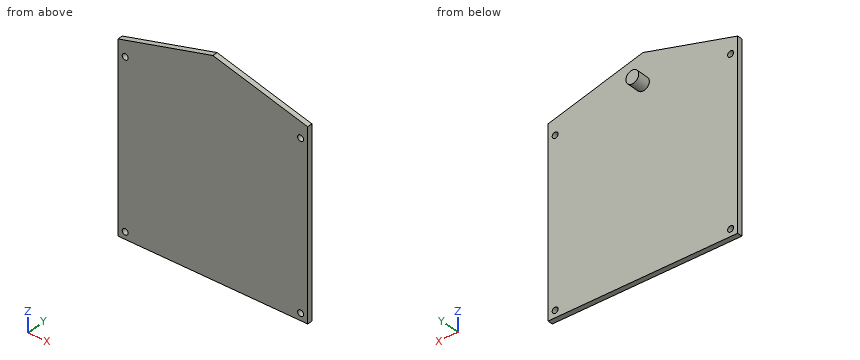
```python
from build123d import *

# Parameters (mm, degrees)
PAD_DEPTH    = 4
SKETCH001_R  = 2.3
POCKET_DEPTH = 5
SKETCH002_R  = 5
PAD001_DEPTH = 10


with BuildPart() as part:
    # Sketch → Pad (new body)
    with BuildSketch(Plane.XZ):
        Polygon((0, 0), (147, 0), (147, 143.135135), (73.5, 163), (0, 143.135135), align=None)
    extrude(amount=PAD_DEPTH)

    # Sketch001 (on Face7 of Pad) → Pocket (cut)
    with BuildSketch(Plane.XZ.offset(4)):
        with Locations((5.5, 5.5)):
            Circle(SKETCH001_R)
        with Locations((141.5, 5.5)):
            Circle(SKETCH001_R)
        with Locations((141.5, 132.5)):
            Circle(SKETCH001_R)
        with Locations((5.5, 132.5)):
            Circle(SKETCH001_R)
    extrude(amount=-POCKET_DEPTH, mode=Mode.SUBTRACT)

    # Sketch002 (on Face4 of Pocket) → Pad001 (join)
    with BuildSketch(Plane(origin=(0, 0, 0), x_dir=(1, 0, 0), z_dir=(0, 1, 0))):
        with Locations((73.5, -140)):
            Circle(SKETCH002_R)
    extrude(amount=PAD001_DEPTH)


solid = part.part
```
Geometry: final body of the model. Coordinates: model frame, mm. Give positions to 0.01 mm unless a question says otherwise; leave off trailing zeros. Loops run counter-clockwise (first coordinate to the right, second up) from the corner with the lowest first, then second, coordinate; pieces in that order, holes last. Notation, with made-up numbers: (-31, 28) - (17, 28) arc R14 ccw to (17, 43) - close; hole circle Ø3 at (52, 37). An arc over 180 degrees is marked (long way). Answer as CSV lines item,"result". Start each with the question number.
(1) Pin query (flat end, axial travel): P1, Ø4, axis at x = 141.5, z = 132.5, coming from the -Y side; P2, Ø2, axis at x = 129, z = 86.5, coming from the +Y side; P3, Ø3, axis at x = 71, y = 1, coming from the +Z side. Return the tip coordinate at first contact, or that it passes through.
(2) Ray query, line 1 along X through (y, z) = (-1.85, 132.5); line 2 along Z through (x, y) = (141.5, -2); line 3 along Y through (x, z) = (15.5, 80.5). Return the intervals inside material, ascending. Write a range as [from, to].
(3) Section query C-C (y = 7.5). Output: boundary loops of the cut face in (x, z).
(4) Section query A-A (z = 132.5). Output: boundary loops of the cut face in (x, y).
(5) Section query B-B (x = 141.5). Output: boundary loops of the cut face in (y, z), and give its area (3 significant figures).
(6) Section query D-D (z = 149). Output: boundary loops of the cut face in (x, y).
Worked answers:
1,P1,"passes through"
1,P2,"stops at y = 0"
1,P3,"stops at z = 162.63"
2,line 1,"x = [0, 3.2], [7.8, 139.2], [143.8, 147]"
2,line 2,"z = [0, 3.2], [7.8, 130.2], [134.8, 144.62]"
2,line 3,"y = [-4, 0]"
3,outline,"circle Ø10 at (73.5, 140)"
4,outline,"(0, -4) - (3.2, -4) - (3.2, 0) - (0, 0) - close; (7.8, -4) - (139.2, -4) - (139.2, 0) - (7.8, 0) - close; (143.8, -4) - (147, -4) - (147, 0) - (143.8, 0) - close"
5,outline,"(-4, 0) - (0, 0) - (0, 3.2) - (-4, 3.2) - close; (-4, 7.8) - (0, 7.8) - (0, 130.2) - (-4, 130.2) - close; (-4, 134.8) - (0, 134.8) - (0, 144.62) - (-4, 144.62) - close"
5,area,"542 mm^2"
6,outline,"(21.7, -4) - (125.3, -4) - (125.3, 0) - (21.7, 0) - close"
